Geometry: final body of the model. Coordinates: model frame, mm. Round coordinates to 2 decimals unless told otherwise and drop trailing zeros. Write each loop counter-clockwise with the first axis right and the second up, starting at its lowest first coordinate (ties: lowest second). Pieces come first, ordered by that corner, then holes.
Autodesk Inventor part; units mm, degrees
ref_plane "YZ Plane" through (0, 0, 0) normal (1, 0, 0) x (0, 1, 0)
ref_plane "XZ Plane" through (0, 0, 0) normal (0, 1, 0) x (-1, 0, 0)
ref_plane "XY Plane" through (0, 0, 0) normal (0, 0, 1) x (1, 0, 0)
sketch "Эскиз1" plane through (0, 0, 0) normal (1, 0, 0) x (0, 1, 0)
  line L0 (0, -42) -> (0, 42) construction
  line L1 (-15, -26) -> (15, -26)
  line L2 (15, -26) -> (15, 26)
  line L3 (15, 26) -> (-15, 26)
  line L4 (-15, 26) -> (-15, -26)
  line L5 (-15, -26) -> (15, 26) construction
  line L6 (15, -26) -> (-15, 26) construction
  line L7 (5, 30) -> (-5, 30)
  line L8 (-5, 30) -> (-5, 26)
  line L9 (-5, 26) -> (5, 26)
  line L10 (5, 26) -> (5, 30)
  line L11 (5, -26) -> (-5, -26)
  line L12 (-5, -26) -> (-5, -30)
  line L13 (-5, -30) -> (5, -30)
  line L14 (5, -30) -> (5, -26)
  point P0 (0, 0)
  dimension "d3" = 30
  dimension "d4" = 60
  dimension "d5" = 4
  dimension "d6" = 10
extrude "Выдавливание1" add sketch "Эскиз1" along normal mid plane 4
properties part number "Кусочек барабана на 3 см"
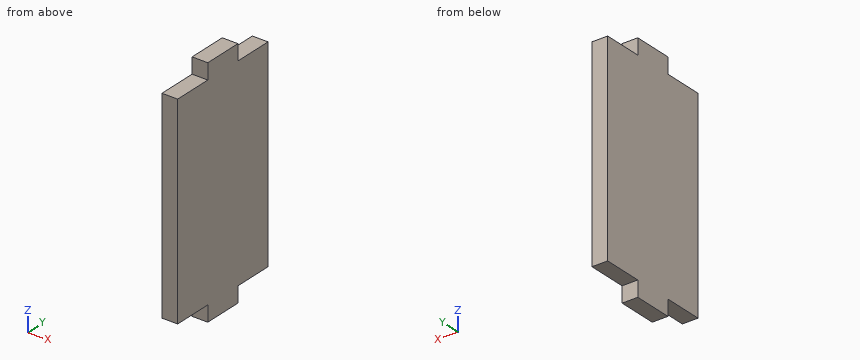
1) Section A-A on x = -0.8. Output: boundary loops of the cut face in (y, z), plus the area to 3 significant figures.
2) Line query: probe 1 along Z at (x, y) = (-1, 12.5). Output: solid intervals per line, ascending.
3) First-contact query: P1, Ø1.2, axis at x = 0.5, y = -9, coming from the +Z side; P2, Ø1.2, axis at x = -1, z = 28, coming from the -Y side; P3, Ø2, axis at x = -1, y = 9.5, coming from the -Z side. Flat tips, straight axial feed; report the tip coordinate or a pass-through.
4) Section B-B on y = -11. Output: boundary loops of the cut face in (x, z).
Filled in:
1. outline: (-15, -26) - (-5, -26) - (-5, -30) - (5, -30) - (5, -26) - (15, -26) - (15, 26) - (5, 26) - (5, 30) - (-5, 30) - (-5, 26) - (-15, 26) - close
1. area: 1,640 mm2
2. probe 1: z = -26 to 26
3. P1: stops at z = 26
3. P2: stops at y = -5
3. P3: stops at z = -26
4. outline: (-2, -26) - (2, -26) - (2, 26) - (-2, 26) - close
